Source: CAD feature listing. Evaluate the final solid. Frame: model axes, mm. Give positions to 0.01 mm unless a question says otherwise; leave off trailing zeros. Order: outer loops, then holes, each group sorted by start corner. A loop starts at its lowest first (then second) coordinate and runs counter-clockwise, first axis right, second up.
1) Section C-C, the plane y = -1.5. Return loops of the section in (x, z) (3 decimals).
2) Section B-B, the plane x = 44.5. Return loops of the section in (y, z) (3 decimals), plus the area to 3 significant figures.
3) First-contact query: P1, Ø1, axis at y = -7, z = 1.5, coming from the -X side; P2, Ø1, axis at y = -39.5, z = 1.5, coming from the -X side; P3, Ø1, axis at y = -2, z = 2, coming from the +X side. Flat tips, straight axial feed; report the tip coordinate or a pass-through.
4) Material intervals for line 1 (X direction, y = -8, z = 2); line 2 (X direction, y = -5, z = 1.15); line 3 (X direction, y = -48, z = 2.55), sorted ascending.
5) Section A-A, the plane y = -29. Give the number of separate pieces and of enclosed holes in the cut face, plus the area to 3 significant figures.
```python
from build123d import *

# Parameters (mm, degrees)
SKETCH1_R           = 2.60777722
SKETCH1_R_2         = 5.242542832
SKETCH1_R_3         = 3.166937391
SKETCH1_R_4         = 9.783190039
SKETCH1_R_5         = 3.439146742
SKETCH1_R_6         = 2.333532814
SKETCH1_R_7         = 1.949356062
BOSS_EXTRUDE1_DEPTH = 3.175


with BuildPart() as part:
    # Sketch1 → Boss-Extrude1 (new body)
    with BuildSketch(Plane.XY):
        with BuildLine():
            Line((-57.15, 0), (-59.69, 0))
            Line((-59.69, 0), (-59.69, -12.7))
            Line((-59.69, -12.7), (-62.981786531, -15.991786531))
            Line((-62.981786531, -15.991786531), (-61.033522603, -17.940050458))
            Line((-61.033522603, -17.940050458), (-57.15, -14.056527855))
            Line((-57.15, -14.056527855), (-57.15, -3.302))
            Line((-57.15, -3.302), (-19.05, -3.302))
            Line((-19.05, -3.302), (-19.05, 0))
            Line((-19.05, 0), (19.05, 0))
            Line((19.05, 0), (19.05, -3.302))
            Line((19.05, -3.302), (57.15, -3.302))
            Line((57.15, -3.302), (57.15, -14.056527855))
            Line((57.15, -14.056527855), (61.033522603, -17.940050458))
            Line((61.033522603, -17.940050458), (62.981786531, -15.991786531))
            Line((62.981786531, -15.991786531), (59.69, -12.7))
            Line((59.69, -12.7), (59.69, 0))
            Line((59.69, 0), (57.15, 0))
            ThreePointArc((57.15, 0), (60.470428387, 8.562338253), (68.695454545, 12.647411782))
            ThreePointArc((68.695454545, 12.647411782), (69.560764803, 6.35), (69.85, 0))
            ThreePointArc((69.85, 0), (51.587643869, -47.092860393), (6.35, -69.560764803))
            Line((6.35, -69.560764803), (6.35, -66.548))
            Line((6.35, -66.548), (-6.35, -66.548))
            Line((-6.35, -66.548), (-6.35, -69.560764803))
            ThreePointArc((-6.35, -69.560764803), (-51.587643869, -47.092860393), (-69.85, 0))
            ThreePointArc((-69.85, 0), (-69.560764803, 6.35), (-68.695454545, 12.647411782))
            ThreePointArc((-68.695454545, 12.647411782), (-60.470428387, 8.562338253), (-57.15, 0))
        make_face()
        with Locations((-51.460707528, -8.761001901)):
            Circle(SKETCH1_R, mode=Mode.SUBTRACT)
        with Locations((-54.068484748, -26.026352242)):
            Circle(SKETCH1_R_2, mode=Mode.SUBTRACT)
        with Locations((-44.460109085, -17.940050458)):
            Circle(SKETCH1_R_3, mode=Mode.SUBTRACT)
        with Locations((-37.959553388, -35.027121669)):
            Circle(SKETCH1_R_4, mode=Mode.SUBTRACT)
        with Locations((-30.458912199, -12.107533279)):
            Circle(SKETCH1_R_5, mode=Mode.SUBTRACT)
        with Locations((-36.126063319, -20.78380941)):
            Circle(SKETCH1_R_6, mode=Mode.SUBTRACT)
        with Locations((-39.459681626, -12.107533279)):
            Circle(SKETCH1_R_7, mode=Mode.SUBTRACT)
        with Locations(Location((37.959553388, -35.027121669, 0), (0, 0, 180))):
            Circle(SKETCH1_R_4, mode=Mode.SUBTRACT)
        with Locations(Location((36.126063319, -20.78380941, 0), (0, 0, 180))):
            Circle(SKETCH1_R_6, mode=Mode.SUBTRACT)
        with Locations(Location((30.458912199, -12.107533279, 0), (0, 0, 180))):
            Circle(SKETCH1_R_5, mode=Mode.SUBTRACT)
        with Locations(Location((39.459681626, -12.107533279, 0), (0, 0, 180))):
            Circle(SKETCH1_R_7, mode=Mode.SUBTRACT)
        with Locations(Location((44.460109085, -17.940050458, 0), (0, 0, 180))):
            Circle(SKETCH1_R_3, mode=Mode.SUBTRACT)
        with Locations(Location((54.068484748, -26.026352242, 0), (0, 0, 180))):
            Circle(SKETCH1_R_2, mode=Mode.SUBTRACT)
        with Locations(Location((51.460707528, -8.761001901, 0), (0, 0, 180))):
            Circle(SKETCH1_R, mode=Mode.SUBTRACT)
        Polygon((0, -12.7), (-16.44651858, -44.588157329), (0, -53.07055318), align=None, mode=Mode.SUBTRACT)
        Polygon((16.44651858, -44.588157329), (2.965479923, -52.923865877), (2.965479923, -59.078158296), (20.758668378, -59.078158296), (20.758668378, -8.761001901), (2.965479923, -8.761001901), (2.965479923, -12.7), align=None, mode=Mode.SUBTRACT)
        Polygon((0, -59.078158296), (-23.268802527, -59.078158296), (-23.268802527, -12.107533279), (-23.268802527, -8.761001901), (0, -8.761001901), (0, -10.43426759), (-20.676383037, -10.43426759), (-20.676383037, -56.497278023), (0, -56.497278023), align=None, mode=Mode.SUBTRACT)
    extrude(amount=BOSS_EXTRUDE1_DEPTH)


solid = part.part
```
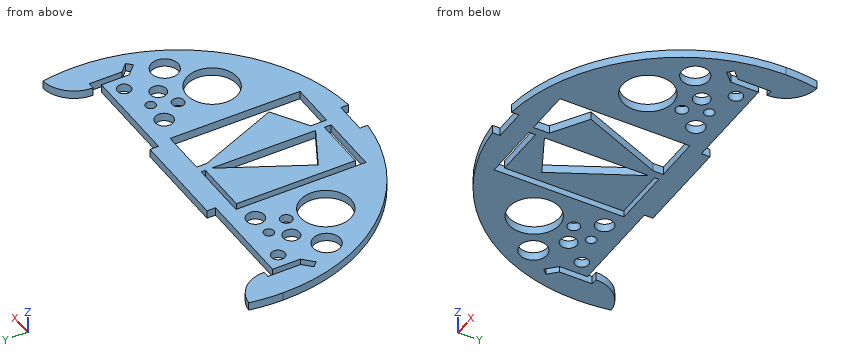
From the geometry:
1. outline: (-69.834, 0) - (-59.69, 0) - (-59.69, 3.175) - (-69.834, 3.175) - close; (-19.05, 0) - (19.05, 0) - (19.05, 3.175) - (-19.05, 3.175) - close; (59.69, 0) - (69.834, 0) - (69.834, 3.175) - (59.69, 3.175) - close
2. outline: (-53.84, 0) - (-42.303, 0) - (-42.303, 3.175) - (-53.84, 3.175) - close; (-27.752, 0) - (-21.107, 0) - (-21.107, 3.175) - (-27.752, 3.175) - close; (-14.773, 0) - (-3.302, 0) - (-3.302, 3.175) - (-14.773, 3.175) - close
2. area: 94.2 mm2
3. P1: stops at x = -69.55
3. P2: stops at x = -57.95
3. P3: stops at x = 69.83
4. line 1: x = -69.39 to -59.69, -57.15 to -53.95, -48.97 to 48.97, 53.95 to 57.15, 59.69 to 69.39
4. line 2: x = -69.67 to -59.69, -57.15 to 57.15, 59.69 to 69.67
4. line 3: x = -50.74 to -23.27, -20.68 to -9.83, 0 to 10.93, 20.76 to 50.74
5. separate pieces: 8
5. enclosed holes: 0
5. area: 181 mm2
